Design review of the part built by this model. Coordinates are the model's own, in mm. A direction names the side the tool comes from. Round coordinates to 2 decimals unless told otherwise and drop trailing zeros. Loops run counter-clockwise (first coordinate to the right, second up) from the corner with the lowest first, then second, coordinate; pieces in that order, holes last. Notation, with made-up numbers: (-7.75, 23) - (50.25, 23) arc R7 ccw to (50.25, 28) - close; hole circle Ø10 at (26.5, -10). An arc over 180 degrees is marked (long way). Use one line per item in the form item = value. Start each with the question number.
(1) We need section C-C, the plane z = 712. Write out the cut boundary in (x, y).
(2) Wall thickness on probe 1 along Y at (x, z) = (526.25, 712); probe 2 along Z at (x, y) = (516.75, -12); probe 3 along X at (y, z) = (-4, 724): over which ranges is each line inside the solid? List them lowest first. Write a range as [from, to].
(3) We need section B-B, the plane z = 698.5. Write out the cut boundary in (x, y).
(4) The part is to be moulded in two halves that separate along Z. For faces 1 (the flat face through (523, -5, 701)), 2 (the cylindrical face through (518.944, -16.558, 730.058)), 3 (the cylindrical face through (518.944, 14.024, 728.815)), say which applies: released by +Z, released by -Z, zero draft, split by the parting line, or undercut.
(5) We need section D-D, the plane x = 518.5. Write out the cut boundary in (y, z) (3 decimals), then the cut area to 3 significant figures.
(6) For pin 1 (4.5 mm diameter, centred on y = -14.14, z = 697.86, fed in from +X); pin 2 (4 mm diameter, centred on x = 525.5, z = 723, fed in from -Y); pin 3 (2 mm diameter, centred on y = -4, z = 712, fed in from +X); pin 4 (6 mm diameter, centred on y = -14.14, z = 726.14, fed in from +X), all flat-tipped, find the tip position at first contact; note any pin that passes through.
(7) We need section A-A, the plane y = 0. Write out the cut boundary in (x, z).
(8) Machinability: for faces 4 (the cylindrical face through (518.944, -14.26, 728.815)), 5 (the cylindrical face through (526.52, -3.95, 713.25)), which of the approach directions +Z, -Z, +X, -X, +Y, -Y give a long, thin tool a straight path to every point of the face, cutting with its end or side? Answer none if there is none.
Autodesk Inventor part; units mm, degrees
ref_plane "Work Plane1" through (515, 0, 712) normal (1, 0, 0) x (0, 0, -1)
ref_plane "YZ Plane" through (0, 0, 0) normal (1, 0, 0) x (0, 1, 0)
ref_plane "XZ Plane" through (0, 0, 0) normal (0, 1, 0) x (-1, 0, 0)
ref_plane "Work Plane1" through (515, 0, 712) normal (1, 0, 0) x (0, 0, -1)
sketch "Sketch1" plane through (515, 0, 712) normal (1, 0, 0) x (0, 0, -1)
  circle A0 centre (0, 0) radius 24.5
  circle A1 centre (0, 0) radius 13.5
  circle A2 centre (14.1421, -14.1421) radius 2.675
  circle A3 centre (14.1421, 14.1421) radius 2.675
  circle A4 centre (-14.1421, 14.1421) radius 2.675
  circle A5 centre (-14.1421, -14.1421) radius 2.675
  arc A6 (-20, 3.5) -> (-20, -3.5) centre (-20, 0) ccw
  arc A7 (-20, -3.5) -> (-20, 3.5) centre (-20, 0) ccw
  point P0 (712, 0)
extrude "Extrusion1" add sketch "Sketch1" along normal blind 8 contours A0 | A1
sketch "Sketch2" plane through (523, 0, 712) normal (1, 0, 0) x (0, 0, -1)
  circle A0 centre (0, 0) radius 11
  point P0 (712, 0)
  dimension "d2" = 22
extrude "Extrusion2" add sketch "Sketch2" along normal blind 5
sketch "Sketch3" plane through (528, 0, 712) normal (1, 0, 0) x (0, 0, -1)
  circle A0 centre (0, -4.0001) radius 1.25
  circle A1 centre (0, 3.9999) radius 1.25
  circle A2 centre (0, 0) radius 11
  point P0 (712, 0)
  dimension "d14" = 8
  dimension "d15" = 22
extrude "Extrusion3" cut sketch "Sketch3" against normal blind 3 contours A0 | A1
properties part number "Herramienta Marcador Base"
Data:
q1.outline = (515, -24.5) - (523, -24.5) - (523, -11) - (528, -11) - (528, -5.25) - (525, -5.25) - (525, -2.75) - (528, -2.75) - (528, 2.75) - (525, 2.75) - (525, 5.25) - (528, 5.25) - (528, 11) - (523, 11) - (523, 24.5) - (515, 24.5) - close
q2.probe_1 = [-11, -5.25], [-2.75, 2.75], [5.25, 11]
q2.probe_2 = [690.64, 696.26], [699.46, 724.54], [727.74, 733.36]
q2.probe_3 = [515, 523]
q3.outline = (515, -20.45) - (523, -20.45) - (523, -16.74) - (515, -16.74) - close; (515, -11.55) - (523, -11.55) - (523, 11.55) - (515, 11.55) - close; (515, 16.74) - (523, 16.74) - (523, 20.45) - (515, 20.45) - close
q4.face_1 = zero draft
q4.face_2 = split by the parting line
q4.face_3 = undercut
q5.outline = circle Ø49 at (0, 712); hole circle Ø5.35 at (-14.142, 697.858); hole circle Ø5.35 at (-14.142, 726.142); hole circle Ø7 at (0, 732); hole circle Ø5.35 at (14.142, 697.858); hole circle Ø5.35 at (14.142, 726.142)
q5.area = 1,760 mm^2
q6.pin_1 = through
q6.pin_2 = -6.32
q6.pin_3 = 525
q6.pin_4 = 523
q7.outline = (515, 687.5) - (523, 687.5) - (523, 701) - (528, 701) - (528, 723) - (523, 723) - (523, 728.5) - (515, 728.5) - close; (515, 735.5) - (523, 735.5) - (523, 736.5) - (515, 736.5) - close
q8.face_4 = +X, -X
q8.face_5 = +X
